Part model, mm, in its own coordinate system. A direction names the side the tool comes from. Round coordinates to 2 decimals unless told otherwise and drop trailing zeros. Order: outer loops, then holes, each group sorted by start corner. A loop starts at its lowest first (then second) coordinate and runs counter-clockwise, first axis right, second up. Notation, with made-up numbers: (53.5, 2.5) -> (70.5, 2.5) arc R7 cw to (70.5, 8.5) -> close; hole circle Ø6 at (1, 11.25). An arc over 180 degrees is marked (long way). Use CSV: the item, a comma, the result in double quotes.
Autodesk Inventor part; units mm, degrees
ref_plane "YZ Plane" through (0, 0, 0) normal (1, 0, 0) x (0, 1, 0)
ref_plane "XZ Plane" through (0, 0, 0) normal (0, 1, 0) x (-1, 0, 0)
ref_plane "XY Plane" through (0, 0, 0) normal (0, 0, 1) x (1, 0, 0)
sketch "Sketch1" plane through (0, 0, 0) normal (0, 1, 0) x (-1, 0, 0)
  line L0 (23.25, 15.71) -> (-23.25, 15.71)
  line L1 (-23.25, 15.71) -> (-23.25, -15.71)
  line L2 (-23.25, -15.71) -> (23.25, -15.71)
  line L3 (23.25, -15.71) -> (23.25, 15.71)
  line L4 (23.25, 15.71) -> (-23.25, -15.71) construction
  line L5 (-23.25, 15.71) -> (23.25, -15.71) construction
  circle A0 centre (20.75, -13.21) radius 1.75
  circle A1 centre (-20.75, 13.21) radius 1.75
  line L6 (14.0587, -12.8063) -> (6.8338, -12.8063)
  line L7 (6.8338, -12.8063) -> (6.8338, -10.1137)
  line L8 (6.8338, -10.1137) -> (14.0587, -10.1137)
  line L9 (14.0587, -10.1137) -> (14.0587, -12.8063)
  line L10 (14.0587, -12.8063) -> (6.8338, -10.1137) construction
  line L11 (6.8338, -12.8063) -> (14.0587, -10.1137) construction
  point P0 (0, 0)
  point P1 (10.4463, -11.46)
  dimension "d0" = 46.5
  dimension "d1" = 31.42
  dimension "d2" = 3.5
  dimension "d3" = 3.5
  dimension "d4" = 2.5
  dimension "d5" = 2.5
  dimension "d6" = 2.5
  dimension "d7" = 2.5
extrude "Extrusion1" add sketch "Sketch1" along normal blind 1.7
extrude "Extrusion2" add sketch "Sketch1" along normal blind 13.25 contours L6 L7 L8 L9
sketch "Sketch2" plane through (0, 1.7, 0) normal (0, 1, 0) x (1, 0, 0)
  line L0 (-8.2019, 1.2171) -> (20.3938, 1.2171) construction
  line L1 (20.3938, 1.2171) -> (20.3938, -2.5127) construction
  line L2 (20.3938, -2.5127) -> (-8.2019, -2.5127) construction
  line L3 (-8.2019, -2.5127) -> (-8.2019, 1.2171) construction
  point P0 (0, 0)
sketch "Sketch3" plane through (23.25, 0, -15.71) normal (0, 0, -1) x (-1, 0, 0)
  point P0 (23.25, 0)
properties part number "Sound Detect"
(1) Cut at B-B, the plane x = -20.75. Give the cut face in (y, z), then the cut area to 3 significant figures.
Reply:
outline,"(0, -15.71) -> (1.7, -15.71) -> (1.7, -14.96) -> (0, -14.96) -> close; (0, -11.46) -> (1.7, -11.46) -> (1.7, 15.71) -> (0, 15.71) -> close"
area,"47.5 mm2"
(2) Drop flat-ended pins along their axis: P1, Ø3, axis at y = 5.5, z = -11.5, coming from the -X side; P2, Ø12, axis at x = -0.5, z = 8.5, coming from the +Y side; P3, Ø2, axis at x = -10, y = 10, coming from the -Z side; P4, Ø5, axis at x = 3, y = 4.5, coming from the -Z side. Give the stop position or say it passes through.
Reply:
P1,"x = -14.06"
P2,"y = 1.7"
P3,"z = -12.81"
P4,"through"
(3) Which spindle directions (+Z, -Z, +X, -X, +Y, -Y) get a long thin tool onto all of the face, cutting with end or side? Do faces 1 (the face through (-10, 7, -12.806)), 2 (the face through (-14.059, 7, -11)), 3 (the face through (-6.834, 7, -11)). Say none if no direction does.
Reply:
face 1,"-Z, +X, -X, +Y"
face 2,"+Z, -Z, -X, +Y"
face 3,"+Z, -Z, +X, +Y"
(4) Cut at D-D, the plane z = -4.5. Give the cut face in (x, y).
Reply:
outline,"(-23.25, 0) -> (23.25, 0) -> (23.25, 1.7) -> (-23.25, 1.7) -> close"
(5) Cut at A-A, the plane z = 13.21. Give the cut face in (x, y), then the cut area to 3 significant figures.
Reply:
outline,"(-23.25, 0) -> (19, 0) -> (19, 1.7) -> (-23.25, 1.7) -> close; (22.5, 0) -> (23.25, 0) -> (23.25, 1.7) -> (22.5, 1.7) -> close"
area,"73.1 mm2"
(6) Probe probe 1 along Z at (x, y) = (20.75, 0.5); probe 2 along Z at (x, y) = (-20.75, 0.8); probe 3 along Y at (x, z) = (-6.5, -13.5). List the from-to ranges inside material, lowest first. Write a range as [from, to].
Reply:
probe 1,"[-15.71, 11.46], [14.96, 15.71]"
probe 2,"[-15.71, -14.96], [-11.46, 15.71]"
probe 3,"[0, 1.7]"
(7) Cut at C-C, the plane x = -8. Give the cut face in (y, z), then the cut area to 3 significant figures.
Reply:
outline,"(0, -15.71) -> (1.7, -15.71) -> (1.7, -12.81) -> (13.25, -12.81) -> (13.25, -10.11) -> (1.7, -10.11) -> (1.7, 15.71) -> (0, 15.71) -> close"
area,"84.5 mm2"
(8) Pull direction Z, two halves, no side cores. Call faces 4 (the face through (-10, 7, -10.114)), 5 (the face through (23.25, 1, 0)), 6 (the face through (22.04, 0.84, 12.03)), 7 (the face through (-19, 0.84, -13.29)): released by +Z, released by -Z, zero draft, split by the parting line, or undercut.
Reply:
face 4,"released by +Z"
face 5,"zero draft"
face 6,"undercut"
face 7,"undercut"
